```python
from build123d import *

# Parameters (mm, degrees)
F0_W     = 200
F0_H     = 100
F1_DEPTH = 120


with BuildPart() as f1:
    # F0 (on Top) → F1 (new body)
    with BuildSketch(Plane.XY):
        Rectangle(F0_W, F0_H)
    extrude(amount=F1_DEPTH)

    # F2 (on face) → F3 (revolve)
    with BuildSketch(Plane.XY.offset(120)):
        with BuildLine():
            Line((60, 30), (60, -30))
            ThreePointArc((60, -30), (90, 0), (60, 30))
        make_face()
    revolve(axis=Axis((60, 0, 120), (0, -1, 0)))

    # F4 (on face) → F7 section 0
    with BuildSketch(Plane(origin=(-100, 0, 0), x_dir=(0, -1, 0), z_dir=(-1, 0, 0))):
        with BuildLine():
            add(Edge.make_bspline(
                [(0, 25), (43.30127, 25), (21.650635, 77.5), (0, 130), (-21.650635, 77.5), (-43.30127, 25), (0, 25)],
                knots=[0, 0, 0, 2.094395, 2.094395, 4.18879, 4.18879, 6.283185, 6.283185, 6.283185], degree=2, weights=[1, 0.5, 1, 0.5, 1, 0.5, 1]))
        make_face()
    # F6 (on offset) → F7 section 1
    with BuildSketch(Plane.YZ.offset(-250)):
        with BuildLine():
            add(Edge.make_bspline(
                [(0, 42.5), (21.650635, 42.5), (10.825318, 68.75), (0, 95), (-10.825318, 68.75), (-21.650635, 42.5), (0, 42.5)],
                knots=[0, 0, 0, 2.094395, 2.094395, 4.18879, 4.18879, 6.283185, 6.283185, 6.283185], degree=2, weights=[1, 0.5, 1, 0.5, 1, 0.5, 1]))
        make_face()
    loft()


solid = f1.part
```
CAD build for the part. Positions are in the model's coordinates, mm. A direction names the side the tool comes from. Round coordinates to 2 decimals unless told otherwise and drop trailing zeros. Loops run counter-clockwise (first coordinate to the right, second up) from the corner with the lowest first, then second, coordinate; pieces in that order, holes last. Notation, with made-up numbers: M 32,88.5 L 61,88.5 A33 ccw 61,121.5 Z; hole C 59,-3.75 d3. An arc over 180 degrees is marked long. Return JSON: item names as keys, results as strings. Group by question number.
(1) Saw through at A-A, the plane y = 35.5. List the corners of the cut face in (x, z).
(2) Drop flat-ended pins along their axis: P1, Ø2, axis at y = -25.5, z = 47, coming from the -X side; P2, Ø6, axis at x = -169, y = 8.5, coming from the +Z side. Give the stop position or say it passes through.
(3) Saw through at B-B, the plane z = 9. List the corners of the cut face in (x, y).
(4) Tool access for faces 1 (the flat face through (100, -1, 59)), 2 (the flat face through (-100, 22, 35)): list every direction of +Z, -Z, +X, -X, +Y, -Y with a clear straight run to the whole face (end or side of a thin tool).
(5) Saw through at C-C, the plane x = 43. List the corners of the cut face in (y, z).
(6) Wall check: probe 1 along Z at (x, y) = (74, 37.5); probe 2 along X at (y, z) = (-24, 80.5); probe 3 along Z at (x, y) = (59.5, 25.5). Give the ranges that are in metal, low to high. Write a range as [from, to].
Answer list:
{
 "1": {"outline": "M -100,0 L 100,0 L 100,120 L -100,120 Z"},
 "2": {"P1": "x = -100", "P2": "z = 85.88"},
 "3": {"outline": "M -100,-50 L 100,-50 L 100,50 L -100,50 Z"},
 "4": {"face 1": "+Z, -Z, +X, +Y, -Y", "face 2": "-X"},
 "5": {"outline": "M -50,0 L 50,0 L 50,120 L 24.72,120 A24.72 ccw -24.72,120 L -50,120 Z"},
 "6": {"probe 1": "[0, 120]", "probe 2": "[-100, 100]", "probe 3": "[0, 135.8]"}
}
